Design review of the part shown in the three views and the two pictorial views. Dimensions are in mm from the part's minimum x, y and z. A direction names the side the tool comes from. Round coordinates to 2 decimals unless told otherwise and drop trailing zeros. Write each loop counter-clockwise with the first axis right and the second up, starting at its lowest first coordinate (ties: lowest second). Pieces come first, ordered by that corner, then holes. Notation, with made-up numbers: (62, 72) -> (83, 72) arc R4 cw to (83, 76) -> close; hole circle Ø4 at (32, 81.5). An arc over 180 degrees is marked (long way). One line per question, with ' | ' between items. Start each with the question number.
1) Consider section C-C (x = 61.5). Give the boundary of the cut face in (y, z).
2) For the marked faces 1 and 2, list the 3-axis set-ups (+Z, -Z, +X, -X, +Y, -Y) from which the entire face can be reached by the end or side of a thin tool; tool diameter is ignored.
3) Consider section D-D (y = 14.25). Give the boundary of the cut face in (x, z).
4) For probe 1 along Z at (x, y) = (20, 22.5); probe 2 along Y at (x, z) = (48.5, 3.5); probe 3 along X at (y, z) = (5.75, 1.5), list the stretches that pass through material, from the lowest coordinate up.
5) Consider section A-A (z = 6.6). Give the boundary of the cut face in (x, y).
6) Consider section B-B (x = 20). Give the boundary of the cut face in (y, z).
7) Insertion check: pin 1 Ø5 at (y, z) = (19, 5) entering from +X; pin 2 Ø3 at (x, y) = (59, 9) entering from +Z; pin 3 Ø3 at (x, z) = (40.5, 2.5) entering from -Y; pin 4 Ø2.5 at (x, z) = (20, 6.6) entering from -Y. Each pin has a flat end and moves straight along its axis. Give the tip position at first contact, or say it passes through.
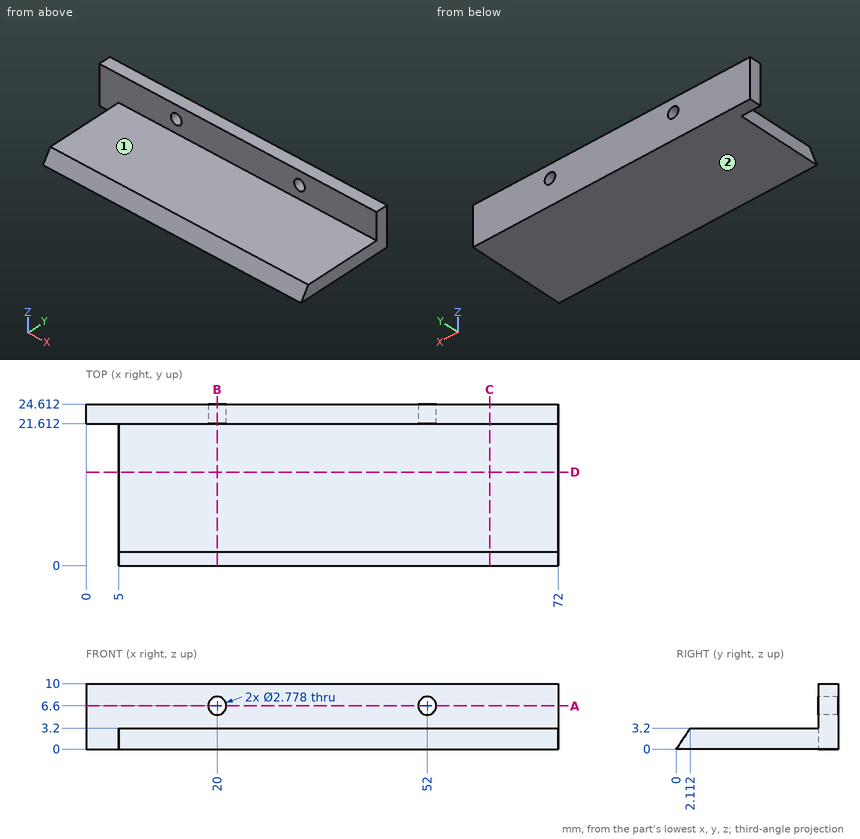
From the geometry:
1) outline: (0, 0) -> (24.61, 0) -> (24.61, 10) -> (21.61, 10) -> (21.61, 3.2) -> (2.11, 3.2) -> close
2) face 1: +Z, +X, -X, -Y | face 2: -Z, +X, -X, +Y, -Y
3) outline: (5, 0) -> (72, 0) -> (72, 3.2) -> (5, 3.2) -> close
4) probe 1: z = 0 to 5.21, 7.99 to 10 | probe 2: y = 21.61 to 24.61 | probe 3: x = 5 to 72
5) outline: (0, 21.61) -> (18.61, 21.61) -> (18.61, 24.61) -> (0, 24.61) -> close; (21.39, 21.61) -> (50.61, 21.61) -> (50.61, 24.61) -> (21.39, 24.61) -> close; (53.39, 21.61) -> (72, 21.61) -> (72, 24.61) -> (53.39, 24.61) -> close
6) outline: (0, 0) -> (24.61, 0) -> (24.61, 5.21) -> (21.61, 5.21) -> (21.61, 3.2) -> (2.11, 3.2) -> close; (21.61, 7.99) -> (24.61, 7.99) -> (24.61, 10) -> (21.61, 10) -> close
7) pin 1: stops at x = 72 | pin 2: stops at z = 3.2 | pin 3: stops at y = 0.66 | pin 4: passes through
